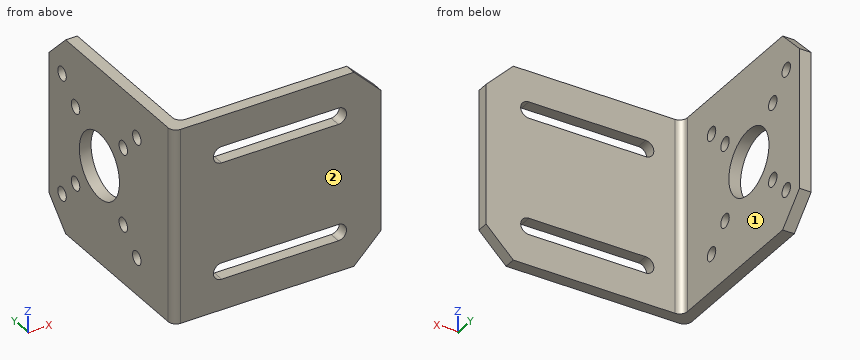
```python
from build123d import *

# Parameters (mm, degrees)
BOSS_EXTRUDE1_DEPTH = 50
SKETCH2_R           = 8.320074994
SKETCH2_R_2         = 1.75
CUT_EXTRUDE1_DEPTH  = 4
CHAMFER1_SIZE       = 7
CHAMFER2_SIZE       = 7
CUT_EXTRUDE2_DEPTH  = 50


with BuildPart() as part:
    # Sketch1 → Boss-Extrude1 (new body)
    with BuildSketch(Plane.XY):
        with BuildLine():
            Line((0, 51.5), (0, 2))
            ThreePointArc((0, 2), (0.585786438, 0.585786438), (2, 0))
            Line((2, 0), (53.5, 0))
            Line((53.5, 0), (53.5, 3))
            Line((53.5, 3), (5, 3))
            ThreePointArc((5, 3), (3.585786438, 3.585786438), (3, 5))
            Line((3, 5), (3, 51.5))
            Line((3, 51.5), (0, 51.5))
        make_face()
    extrude(amount=BOSS_EXTRUDE1_DEPTH)

    # Sketch2 → Cut-Extrude1 (cut, through all)
    with BuildSketch(Plane(origin=(3, 0, 0), x_dir=(0, 0, -1), z_dir=(1, 0, 0))):
        with Locations((-25, 30.5)):
            Circle(SKETCH2_R)
        with Locations((-34.899494937, 40.399494937)):
            Circle(SKETCH2_R_2)
        with Locations((-15.100505063, 40.399494937)):
            Circle(SKETCH2_R_2)
        with Locations((-15.100505063, 20.600505063)):
            Circle(SKETCH2_R_2)
        with Locations((-34.899494937, 20.600505063)):
            Circle(SKETCH2_R_2)
        with Locations((-40.5, 46)):
            Circle(SKETCH2_R_2)
        with Locations((-9.5, 46)):
            Circle(SKETCH2_R_2)
        with Locations((-40.5, 15)):
            Circle(SKETCH2_R_2)
        with Locations((-9.5, 15)):
            Circle(SKETCH2_R_2)
    extrude(amount=-CUT_EXTRUDE1_DEPTH, mode=Mode.SUBTRACT)

    # Chamfer1
    chamfer1_edges = [part.edges().sort_by_distance(p)[0] for p in [
        (1.5, 51.5, 0),
    ]]
    chamfer(chamfer1_edges, length=CHAMFER1_SIZE)

    # Chamfer2
    chamfer2_edges = [part.edges().sort_by_distance(p)[0] for p in [
        (53.5, 1.5, 50),
        (1.5, 51.5, 50),
        (53.5, 1.5, 0),
    ]]
    chamfer(chamfer2_edges, length=CHAMFER2_SIZE)

    # Sketch5 → Cut-Extrude2 (cut)
    with BuildSketch(Plane(origin=(0, 3, 0), x_dir=(1, 0, 0), z_dir=(0, 1, 0))):
        with BuildLine():
            Line((12.5, -7.9), (42.5, -7.9))
            ThreePointArc((42.5, -7.9), (44.6, -10), (42.5, -12.1))
            Line((42.5, -12.1), (12.5, -12.1))
            ThreePointArc((12.5, -12.1), (10.4, -10), (12.5, -7.9))
        make_face()
        with BuildLine():
            Line((12.5, -42.1), (42.5, -42.1))
            ThreePointArc((42.5, -42.1), (44.6, -40), (42.5, -37.9))
            Line((42.5, -37.9), (12.5, -37.9))
            ThreePointArc((12.5, -37.9), (10.4, -40), (12.5, -42.1))
        make_face()
    extrude(amount=-CUT_EXTRUDE2_DEPTH, mode=Mode.SUBTRACT)


solid = part.part
```
Part model, mm, in its own coordinate system. Face numbers are marked on the shaded views. A direction names the side the tool comes from. Coordinates: 2 decimals unless noted, no trailing zeros. Order: outer loops, then holes, each group sorted by start corner. A loop starts at its lowest first (then second) coordinate and runs counter-clockwise, first axis right, second up. Notation, with made-up numbers: (-4.5, 52.5) -> (43.5, 52.5) arc R24 ccw to (43.5, 75.5) -> close; hole circle Ø6 at (70.25, 84). An arc over 180 degrees is marked (long way). Put each result on its own line as item: value. Start each with the question number.
(1) Which spindle directions (+Z, -Z, +X, -X, +Y, -Y) get a long thin tool onto all of the face, cutting with end or side? Do the marked faces 1 and 2. Say none if no direction does.
(2) Band-saw the part on B-B (y = 30.5). Give the cut face in (x, z).
(3) Probe line 1 along Y through (x, z) = (2.1, 40.5); line 2 along Y through (x, z) = (1.2, 9.5); line 3 along Y through (x, z) = (7.5, 6.5). List the from-to ranges inside material, lowest first. Write a range as [from, to].
(4) Band-saw the part on D-D (z = 30). Give the cut face in (x, y), then the cut area to 3 significant figures.
(5) Pin check, flat tips, straight feed: pin 1 Ø6 at (x, z) = (29.5, 24) entering from +Y; pin 2 Ø4.5 at (y, z) = (40.4, 15.1) entering from +X. Stop position of each tip, or through.
(6) Band-saw the part on A-A (x = 18.5). Give the cut face in (y, z).
(7) Band-saw the part on C-C (y = 46). Give the cut face in (x, z).
Determined:
1. face 1: +Z, -Z, +X, +Y
1. face 2: +Z, -Z, +X, -X, -Y
2. outline: (0, 0) -> (3, 0) -> (3, 16.68) -> (0, 16.68) -> close; (0, 33.32) -> (3, 33.32) -> (3, 50) -> (0, 50) -> close
3. line 1: y = [0, 13.25], [16.75, 44.25], [47.75, 51.5]
3. line 2: y = [0.17, 13.25], [16.75, 44.25], [47.75, 51.5]
3. line 3: y = [0, 3]
4. outline: (0, 2) arc R2 ccw to (2, 0) -> (53.5, 0) -> (53.5, 3) -> (5, 3) arc R2 cw to (3, 5) -> (3, 23.85) -> (0, 23.85) -> close; (0, 37.15) -> (3, 37.15) -> (3, 51.5) -> (0, 51.5) -> close
4. area: 266 mm²
5. pin 1: stops at y = 3
5. pin 2: stops at x = 3
6. outline: (0, 0) -> (3, 0) -> (3, 7.9) -> (0, 7.9) -> close; (0, 12.1) -> (3, 12.1) -> (3, 37.9) -> (0, 37.9) -> close; (0, 42.1) -> (3, 42.1) -> (3, 50) -> (0, 50) -> close
7. outline: (0, 1.5) -> (3, 1.5) -> (3, 7.75) -> (0, 7.75) -> close; (0, 11.25) -> (3, 11.25) -> (3, 38.75) -> (0, 38.75) -> close; (0, 42.25) -> (3, 42.25) -> (3, 48.5) -> (0, 48.5) -> close
